Geometry: final body of the model. Coordinates: model frame, mm. Face numbers are marked on the shaded views. A direction names the side the tool comes from. Round coordinates to 2 decimals unless told otherwise and drop trailing zeros. Write each loop counter-clockwise with the first axis right and the second up, starting at its lowest first coordinate (ties: lowest second). Pieces come first, ordered by that corner, then holes.
from build123d import *

# Parameters (mm, degrees)
PAD_DEPTH       = 10
SKETCH001_R     = 2.2
POCKET_DEPTH    = 76.001
SKETCH002_R     = 4.4
POCKET001_DEPTH = 72.001
FILLET_R        = 1


with BuildPart() as part:
    # Sketch → Pad (new body, symmetric)
    with BuildSketch(Plane.XZ):
        with BuildLine():
            Line((5, 30), (5, 22))
            Line((5, 22), (71, 22))
            Line((71, 22), (71, 30))
            Line((71, 30), (76, 30))
            Line((76, 30), (76, 14))
            Line((38.674177, 3.998576), (76, 14))
            ThreePointArc((38.674177, 3.998576), (19.66843, -8.553267), (12, -30))
            Line((12, -30), (0, -30))
            Line((0, -30), (0, 30))
            Line((0, 30), (5, 30))
        make_face()
    extrude(amount=PAD_DEPTH, both=True)

    # Sketch001 → Pocket (cut, through all)
    with BuildSketch(Plane.YZ):
        with Locations((0, 3.998576)):
            Circle(SKETCH001_R)
        with Locations((0, -19.998576)):
            Circle(SKETCH001_R)
    extrude(amount=POCKET_DEPTH, mode=Mode.SUBTRACT)

    # Sketch002 → Pocket001 (cut, through all)
    with BuildSketch(Plane.YZ.offset(4)):
        with Locations((0, 3.998576)):
            Circle(SKETCH002_R)
        with Locations((0, -19.998576)):
            Circle(SKETCH002_R)
    extrude(amount=POCKET001_DEPTH, mode=Mode.SUBTRACT)

    # Fillet
    fillet_edges = [part.edges().sort_by_distance(p)[0] for p in [
        (76, 0, 30),
        (76, 0, 14),
        (76, 10, 22),
        (76, -10, 22),
        (73.5, -10, 30),
        (73.5, 10, 30),
        (19.66843, -10, -8.553267),
        (19.66843, 10, -8.553267),
        (12, 0, -30),
        (6, -10, -30),
        (6, 10, -30),
        (2.5, 10, 30),
        (2.5, -10, 30),
        (5, 0, 30),
        (71, 0, 30),
    ]]
    fillet(fillet_edges, radius=FILLET_R)


with BuildPart() as part_1:
    # Body placement: moved
    add(part.part.moved(Location((0, -15, 0))))


solid = part_1.part
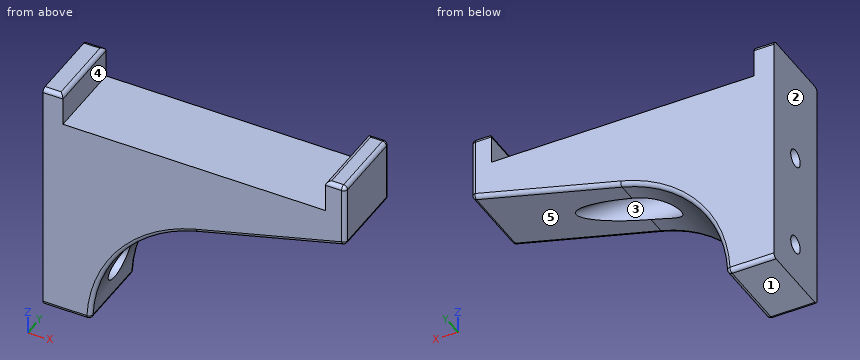
1) Reachability of the marked faces 4 and 5 from +Z, -Z, +X, -X, +Y, -Y: full face, straight path, thin tool, end or side. Return the list, or none.
2) First-contact query: P1, Ø2.5, axis at y = -14, z = -20, coming from the +X side; P2, Ø3, axis at x = 53, y = -20, coming from the +Z side; P3, Ø1, axis at x = 51, y = -11.5, coming from the -Z side. Flat tips, straight axial feed; report the tip coordinate or a pass-through.
3) Section C-C on x = 6. Output: boundary loops of the cut face in (y, z), plus the area to 3 significant figures.
4) Section B-B on y = -9.5. Output: boundary loops of the cut face in (x, z), plus the area to 3 significant figures.
5) Line query: probe 1 along Z at (x, y) = (3, -15); probe 2 along Z at (x, y) = (8.5, -15); probe 3 along X at (y, z) = (-21.5, 23.5). Output: solid intervals per line, ascending.
6) Draft query along Z for the marked faces 1, 2 and 3. Return one class per face: pulls with the +Z half, pulls with the -Z half, needs draft (parallel to the pull), parting line crosses it, or undercut.
7) Section A-A on y = -15. State how many separate pieces and enclosed holes the cut face has, plus the area to 3 significant figures.
Filled in:
1. face 4: +Z, +Y, -Y
1. face 5: -Z, +X, +Y, -Y
2. P1: stops at x = 4
2. P2: stops at z = 22
2. P3: stops at z = 7.17
3. outline: (-25, -29) arc R1 ccw to (-24, -30) - (-6, -30) arc R1 ccw to (-5, -29) - (-5, 22) - (-25, 22) - close; hole circle Ø8.8 at (-15, -20); hole circle Ø8.8 at (-15, 4)
3. area: 918 mm2
4. outline: (0, -30) - (11.03, -30) arc R1 ccw to (12.03, -29.05) arc R36 cw to (38.67, 4) - (75.26, 13.8) arc R1 ccw to (76, 14.77) - (76, 29) arc R1 ccw to (75, 30) - (72, 30) arc R1 ccw to (71, 29) - (71, 22) - (5, 22) - (5, 29) arc R1 ccw to (4, 30) - (0, 30) - close
4. area: 1,910 mm2
5. probe 1: z = -30 to -22.2, -17.8 to 1.8, 6.2 to 30
5. probe 2: z = -30 to -24.4, -15.6 to -0.4, 8.4 to 22
5. probe 3: x = 0 to 5, 71 to 76
6. face 1: pulls with the -Z half
6. face 2: needs draft
6. face 3: undercut
7. separate pieces: 3
7. enclosed holes: 0
7. area: 1,470 mm2
